Part print with two shaded views. Sizes in mm from the minimum x, y, z corner. Give positions to 0.01 mm unless a question says otherwise; leave off trailing zeros. Order: outer loops, then holes, each group sorted by start corner. A loop starts at its lowest first (then second) coordinate and runs counter-clockwise, first axis right, second up. Notation, with made-up numbers: M 4,-30 L 29,-30 A16 cw 29,-23 Z; hole C 27,86.25 d7. An arc over 180 degrees is marked long. Return JSON: item names as keys, results as strings.
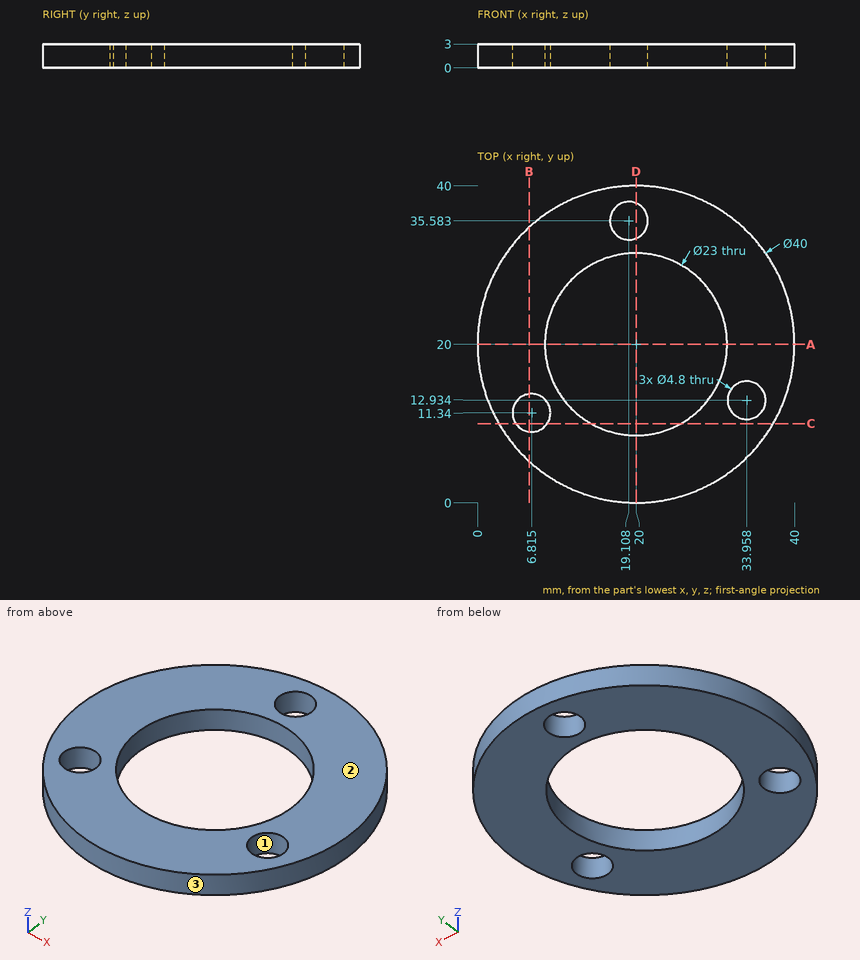
Q1. Pin check, flat tips, straight feed: pin 1 (1 mm diameter, centred on x = 31.5, z = 1, fed in from -Y); pin 2 (4 mm diameter, centred on x = 33.96, y = 12.93, fed in from -Z); pin 3 (1 mm diameter, centred on x = 20.5, z = 2, fed in from +Y). Stop position of each tip, or through.
Established:
{"pin 1": "stops at y = 3.3", "pin 2": "passes through", "pin 3": "stops at y = 40"}
Q2. Probe line 1 along X through (y, z) = (10, 1.3) (1 decimal); line 2 along Y through (x, z) = (25, 1.3) (1 decimal); line 3 along Y through (x, z) = (7, 1.25) (1 decimal). List the from-to ranges inside material, lowest first.
Established:
{"line 1": "x = 2.7 to 4.8, 8.8 to 14.3, 25.7 to 37.3", "line 2": "y = 0.6 to 9.6, 30.4 to 39.4", "line 3": "y = 4.8 to 8.9, 13.7 to 35.2"}
Q3. Band-saw the part on C-C (y = 10). Give the cut face in (x, z).
Established:
{"outline": "M 2.68,0 L 4.82,0 L 4.82,3 L 2.68,3 Z; M 8.81,0 L 14.32,0 L 14.32,3 L 8.81,3 Z; M 25.68,0 L 37.32,0 L 37.32,3 L 25.68,3 Z"}
Q4. Band-saw the part on D-D (x = 20). Give the cut face in (y, z) (1 decimal).
Established:
{"outline": "M 0,0 L 8.5,0 L 8.5,3 L 0,3 Z; M 31.5,0 L 33.4,0 L 33.4,3 L 31.5,3 Z; M 37.8,0 L 40,0 L 40,3 L 37.8,3 Z"}
Q5. Band-saw the part on B-B (x = 6.5). Give the cut face in (y, z).
Established:
{"outline": "M 5.24,0 L 8.96,0 L 8.96,3 L 5.24,3 Z; M 13.72,0 L 34.76,0 L 34.76,3 L 13.72,3 Z"}
Q6. Band-saw the part on A-A (y = 20). Give the cut face in (x, z).
Established:
{"outline": "M 0,0 L 8.5,0 L 8.5,3 L 0,3 Z; M 31.5,0 L 40,0 L 40,3 L 31.5,3 Z"}
Q7. Two-plate mould, pull along X, no slides. Class the marked faces 1, 2 and 3: +X half, -X half, draft (parallel to the pull), parting line (faces both ways), or undercut.
Established:
{"face 1": "undercut", "face 2": "draft", "face 3": "parting line"}
